```python
from build123d import *

# Parameters (mm, degrees)
SKETCH_1_R          = 6
SKETCH_1_R_2        = 4.5
EXTRUDE_1_DEPTH     = 26.5
CUT_EXTRUDE_START   = -1
SKETCH_2_R          = 6
SKETCH_2_R_2        = 5.5
CUT_EXTRUDE_1_DEPTH = 1


with BuildPart() as part:
    # Эскиз1 → Бобышка-Вытянуть1 (new body, symmetric)
    with BuildSketch(Plane.XY):
        Circle(SKETCH_1_R)
        Circle(SKETCH_1_R_2, mode=Mode.SUBTRACT)
    extrude(amount=EXTRUDE_1_DEPTH, both=True)

    # Эскиз2 → Вырез-Вытянуть1 (cut)
    with BuildSketch(Plane.XY.offset(26.5).offset(CUT_EXTRUDE_START)):
        Circle(SKETCH_2_R)
        Circle(SKETCH_2_R_2, mode=Mode.SUBTRACT)
    cut_extrude_1 = extrude(amount=-CUT_EXTRUDE_1_DEPTH, mode=Mode.SUBTRACT)

    # Зеркальное отражение1: Вырез-Вытянуть1 across plane
    add(cut_extrude_1.mirror(Plane.XY), mode=Mode.SUBTRACT)


solid = part.part
```
Geometry: final body of the model. Coordinates: model frame, mm. A direction names the side the tool comes from. Round coordinates to 2 decimals unless told otherwise and drop trailing zeros. Write each loop counter-clockwise with the first axis right and the second up, starting at its lowest first coordinate (ties: lowest second). Pieces come first, ordered by that corner, then holes. Notation, with made-up numbers: (51, 37) -> (64, 37) arc R29 cw to (64, 73) -> close; hole circle Ø6 at (39.5, 39). An arc over 180 degrees is marked (long way). Return JSON: item names as keys, results as strings.
Q1. Mould query, pull axis X, two halves, no side actions, for faces 3 (the cylindrical face through (-1.19, -5.37, -25.01)), 4 (the cylindrical face through (-0.59, 4.46, -0.37)), 5 (the flat face through (3, -5, 25.5)). Classes: +X half, -X half, draft (parallel to the pull), parting line (faces both ways), or undercut.
From the geometry:
{"face 3": "parting line", "face 4": "undercut", "face 5": "draft"}
Q2. Set-up query: faces 1 (the cylindrical face through (-6, 0, 0)), 2 (the cylindrical face through (-1.19, -5.37, 25.01)). Return all of +Z, -Z, +X, -X, +Y, -Y with unobstructed straight access to the full face (end or side cutting, diameter ignored); none if empty.
From the geometry:
{"face 1": "+Z, -Z", "face 2": "none"}
Q3. Ray query, line 1 (Y direction, x = 0, z = 15.5); line 2 (X direction, y = 2.25, z = 9.5); line 3 (Y direction, x = -1.5, z = 23.5). Return the intervals inside material, ascending.
From the geometry:
{"line 1": "-6 to -4.5, 4.5 to 6", "line 2": "-5.56 to -3.9, 3.9 to 5.56", "line 3": "-5.81 to -4.24, 4.24 to 5.81"}
Q4. Section D-D on x = 5. Return the cut outline in (y, z), and give its area (3 significant figures).
From the geometry:
{"outline": "(-3.32, -26.5) -> (3.32, -26.5) -> (3.32, -25.5) -> (2.29, -25.5) -> (2.29, -24.5) -> (3.32, -24.5) -> (3.32, 24.5) -> (2.29, 24.5) -> (2.29, 25.5) -> (3.32, 25.5) -> (3.32, 26.5) -> (-3.32, 26.5) -> (-3.32, 25.5) -> (-2.29, 25.5) -> (-2.29, 24.5) -> (-3.32, 24.5) -> (-3.32, -24.5) -> (-2.29, -24.5) -> (-2.29, -25.5) -> (-3.32, -25.5) -> close", "area": "347 mm2"}
Q5. First-contact query: pin 1 Ø3 at (x, z) = (-4.5, 20) entering from +Y; pin 2 Ø6 at (y, z) = (4.5, 18) entering from -X; pin 3 Ø2 at (x, z) = (4.5, 18) entering from +Y. Flat tips, straight axial feed; report the tip coordinate or a pass-through.
From the geometry:
{"pin 1": "y = 5.2", "pin 2": "x = -5.81", "pin 3": "y = 4.87"}
Q6. Section C-C on z = -2.5. Return the cut outline in (x, y).
From the geometry:
{"outline": "circle Ø12 at (0, 0); hole circle Ø9 at (0, 0)"}
Q7. Section A-A on x = 0. Return the cut outline in (y, z), and give its area (3 significant figures).
From the geometry:
{"outline": "(-6, -26.5) -> (-4.5, -26.5) -> (-4.5, 26.5) -> (-6, 26.5) -> (-6, 25.5) -> (-5.5, 25.5) -> (-5.5, 24.5) -> (-6, 24.5) -> (-6, -24.5) -> (-5.5, -24.5) -> (-5.5, -25.5) -> (-6, -25.5) -> close; (4.5, -26.5) -> (6, -26.5) -> (6, -25.5) -> (5.5, -25.5) -> (5.5, -24.5) -> (6, -24.5) -> (6, 24.5) -> (5.5, 24.5) -> (5.5, 25.5) -> (6, 25.5) -> (6, 26.5) -> (4.5, 26.5) -> close", "area": "157 mm2"}
